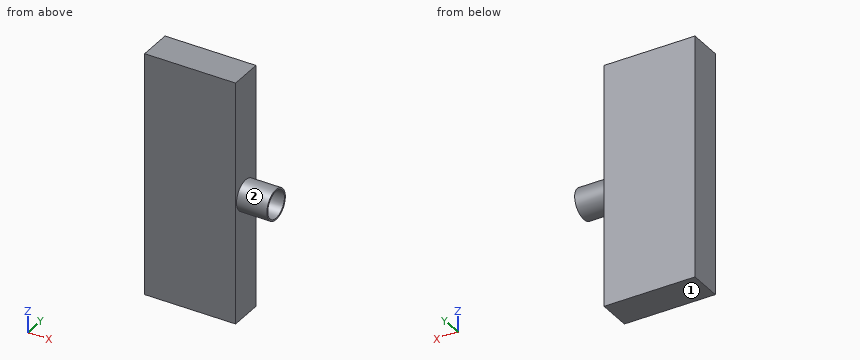
from build123d import *

# Parameters (mm, degrees)
F0_R     = 6.35
F1_DEPTH = 12.7
F2_W     = 13.97
F2_H     = 101.6
F3_DEPTH = 38.1
F4_R     = 5.715
F5_DEPTH = 12.7


with BuildPart() as f1:
    # F0 (on Right) → F1 (new body)
    with BuildSketch(Plane.YZ):
        Circle(F0_R)
    extrude(amount=-F1_DEPTH)

    # F2 (on face) → F3 (join)
    with BuildSketch(Plane(origin=(-12.7, 0, 0), x_dir=(0, -1, 0), z_dir=(-1, 0, 0))):
        Rectangle(F2_W, F2_H)
    extrude(amount=F3_DEPTH)

    # F4 (on face) → F5 (cut)
    with BuildSketch(Plane.YZ):
        Circle(F4_R)
    extrude(amount=-F5_DEPTH, mode=Mode.SUBTRACT)


solid = f1.part
Can you work these out from the model? Positions are in its coordinate system, mm. Face numbers are marked on the shaded views. A direction names the side the tool comes from. Give positions to 0.01 mm unless a question says otherwise; leave off trailing zeros. Loops run counter-clockwise (first coordinate to the right, second up) from the corner with the lowest first, then second, coordinate; pieces in that order, holes last. Notation, with made-up numbers: (74, 36.25) - (97, 36.25) arc R13 ccw to (97, 61.25) - close; hole circle Ø6 at (50.25, 2). An arc over 180 degrees is marked (long way). One line per item, written item: value.
(1) I'm going to push a flat-ended pin straight in: pin 1 (1.5 mm diameter, centred on y = 0, z = -19, fed in from +X). Where does the tip first touch, or does it pass through?
Verdict:
pin 1: x = -12.7
(2) If we section it at A-A, the plane z = 0: List the corners of the cut face in (x, y) for me (3 decimals), plus the area to 3 significant figures.
Verdict:
outline: (-50.8, -6.985) - (-12.7, -6.985) - (-12.7, -6.35) - (0, -6.35) - (0, -5.715) - (-12.7, -5.715) - (-12.7, 5.715) - (0, 5.715) - (0, 6.35) - (-12.7, 6.35) - (-12.7, 6.985) - (-50.8, 6.985) - close
area: 548 mm^2
(3) I need wall thicknesses on line 1 along Z through (x, y) = (-2.5, 0) (3 decimals); line 2 along X through (y, z) = (5.75, -29.5); line 3 along Z through (x, y) = (-4.5, 2.75). Which ranges of each line are inside material? Lowest first, please.
Verdict:
line 1: -6.35 to -5.715, 5.715 to 6.35
line 2: -50.8 to -12.7
line 3: -5.72 to -5.01, 5.01 to 5.72
(4) On a 3-axis mill with a long thin cutter (end or side, diameter ignored), from which of +Z, -Z, +X, -X, +Y, -Y can I reach the whole of each face in a straight line? I mean the marked faces 1 and 2. Say none if no direction works.
Verdict:
face 1: -Z, +X, -X, +Y, -Y
face 2: +X
(5) If we section it at B-B, the plane y = 0: List the corners of the cut face in (x, z) for me (3 decimals).
Verdict:
outline: (-50.8, -50.8) - (-12.7, -50.8) - (-12.7, -6.35) - (0, -6.35) - (0, -5.715) - (-12.7, -5.715) - (-12.7, 5.715) - (0, 5.715) - (0, 6.35) - (-12.7, 6.35) - (-12.7, 50.8) - (-50.8, 50.8) - close
(6) If we section it at D-D, the plane z = 28: List the corners of the cut face in (x, y) for me (3 decimals), plus the area to 3 significant figures.
Verdict:
outline: (-50.8, -6.985) - (-12.7, -6.985) - (-12.7, 6.985) - (-50.8, 6.985) - close
area: 532 mm^2
(7) If we section it at C-C, the plane x = -10.5: List the corners of the cut face in (y, z) for me (3 decimals), plus the area to 3 significant figures.
Verdict:
outline: circle Ø12.7 at (0, 0); hole circle Ø11.43 at (0, 0)
area: 24.1 mm^2
